Could you check a few things on this model? Use its own coordinates, in mm. A direction names the side the tool comes from. Give positions to 0.01 mm unless a question says otherwise; leave off trailing zeros. Order: outer loops, then holes, each group sorted by start corner. A loop starts at its lowest first (then second) coordinate and runs counter-clockwise, first axis right, second up. Notation, with made-up numbers: (75.5, -39.75) -> (94.5, -39.75) arc R34 ccw to (94.5, -0.75) -> close; hole circle Ø8 at (24, -16.75). An arc over 180 degrees is marked (long way). Write each question's results on one line, items separated by ' | '.
```python
from build123d import *

# Parameters (mm, degrees)
F1_DEPTH = 1.5


with BuildPart() as f1:
    # F0 (on Top) → F1 (new body)
    with BuildSketch(Plane.XY):
        with BuildLine():
            Line((30, 15), (-30, 15))
            ThreePointArc((-30, 15), (-33.535534, 13.535534), (-35, 10))
            Line((-35, 10), (-35, 5.638967))
            Line((-35, 5.638967), (-35, -5.509344))
            Line((-35, -5.509344), (-35, -10))
            ThreePointArc((-35, -10), (-33.535534, -13.535534), (-30, -15))
            Line((-30, -15), (30, -15))
            ThreePointArc((30, -15), (33.535534, -13.535534), (35, -10))
            Line((35, -10), (35, -5.509344))
            Line((35, -5.509344), (35, 5.638967))
            Line((35, 5.638967), (35, 10))
            ThreePointArc((35, 10), (33.535534, 13.535534), (30, 15))
        make_face()
        Polygon((-35, -5.509344), (-35, 5.638967), (-48.147307, 10.48606), (-44.754342, 4.34641), (-55.579518, 1.761294), (-44.915912, -2.924228), (-51.701845, -11.325855), align=None)
        Polygon((46.192096, 13.394315), (35, 5.638967), (35, -5.509344), (50.877613, -10.356436), (43.768549, -2.277949), (54.255958, 2.424591), (43.930118, 5.315828), align=None)
    extrude(amount=F1_DEPTH)


solid = f1.part
```
Q1. Suppose I cut it at B-B on z = 1.05. Please give me the cut outline in (x, y), and give its area (3 significant figures).
Here are the results:
outline: (-55.58, 1.76) -> (-44.92, -2.92) -> (-51.7, -11.33) -> (-35, -5.51) -> (-35, -10) arc R5 ccw to (-30, -15) -> (30, -15) arc R5 ccw to (35, -10) -> (35, -5.51) -> (50.88, -10.36) -> (43.77, -2.28) -> (54.26, 2.42) -> (43.93, 5.32) -> (46.19, 13.39) -> (35, 5.64) -> (35, 10) arc R5 ccw to (30, 15) -> (-30, 15) arc R5 ccw to (-35, 10) -> (-35, 5.64) -> (-48.15, 10.49) -> (-44.75, 4.35) -> close | area: 2,500 mm²
Q2. I'm going to push flat-ended pins straight in: pin 1 Ø0.8 at (y, z) = (-7, 1) entering from -X; pin 2 Ø5 at (x, y) = (3, 11) entering from -Z; pin 3 Ø2 at (x, y) = (-36, 12) entering from -Z. Where does each tip first touch, or does it pass through?
Here are the results:
pin 1: stops at x = -48.53 | pin 2: stops at z = 0 | pin 3: passes through
Q3. Suppose I cut it at A-A on y = 7.5. Please give me the cut outline in (x, z), and give its area (3 significant figures).
Here are the results:
outline: (-46.5, 0) -> (-40.05, 0) -> (-40.05, 1.5) -> (-46.5, 1.5) -> close; (-35, 0) -> (35, 0) -> (35, 1.5) -> (-35, 1.5) -> close; (37.69, 0) -> (44.54, 0) -> (44.54, 1.5) -> (37.69, 1.5) -> close | area: 125 mm²
Q4. I need wall thicknesses on line 1 along X through (y, z) = (12, 0.45); line 2 along Y through (x, z) = (47.5, 1.3); line 3 along Y through (x, z) = (-49, 0.3). Which ranges of each line are inside material? Lowest first, please.
Here are the results:
line 1: x = -34.58 to 34.58, 44.18 to 45.8 | line 2: y = -9.33 to -6.52, -0.6 to 4.32 | line 3: y = -10.38 to -7.98, -1.13 to 3.33
Q5. Suppose I cut it at C-C on y = -1. Please give me the cut outline in (x, z), and give its area (3 significant figures).
Here are the results:
outline: (-49.3, 0) -> (46.62, 0) -> (46.62, 1.5) -> (-49.3, 1.5) -> close | area: 144 mm²
Q6. For faces 5 (the flat face through (48.94, 0.04, 0.74)), 6 (the flat face through (-41.48, 8.03, 0.74)), 7 (the flat face through (-50.091, 3.072, 0.74)), which set-ups out of +Z, -Z, +X, -X, +Y, -Y let a thin tool reach every point of the face, with its end or its side?
Here are the results:
face 5: +Z, -Z, +X | face 6: +Z, -Z, +Y | face 7: +Z, -Z, -X
Q7. Thinking about a two-plate mould opening in Y: for faces 1 (the flat face through (40.67, 9.57, 0.74)), 2 (the flat face through (-43.47, -8.46, 0.74)), 3 (the flat face through (-50.32, -0.55, 0.74)), 4 (the flat face through (-1, 0, 1.5)), which applies, +Y half, -Y half, draft (parallel to the pull), parting line (faces both ways), or undercut?
Here are the results:
face 1: +Y half | face 2: -Y half | face 3: undercut | face 4: draft
